```python
from build123d import *

# Parameters (mm, degrees)
SKETCH1_R      = 0.55
EXTRUDE1_DEPTH = 1


with BuildPart() as part:
    # Sketch1 → Extrude1 (new body)
    with BuildSketch(Plane.XY):
        with BuildLine():
            Line((1.656441889, -6.181925288), (2.174079979, -8.113776941))
            ThreePointArc((2.174079979, -8.113776941), (4.904287135, -6.819675043), (7, -4.643274706))
            Line((7, -4.643274706), (7, -3.161966685))
            ThreePointArc((7, -3.161966685), (0, 8.4), (-7, -3.161966685))
            Line((-7, -3.161966685), (-7, -4.643274706))
            ThreePointArc((-7, -4.643274706), (-4.904287135, -6.819675043), (-2.174079979, -8.113776941))
            Line((-2.174079979, -8.113776941), (-1.656441889, -6.181925288))
            ThreePointArc((-1.656441889, -6.181925288), (0, 6.4), (1.656441889, -6.181925288))
        make_face()
        with Locations((-2.86, -6.809962004)):
            Circle(SKETCH1_R, mode=Mode.SUBTRACT)
        with Locations(Location((2.86, -6.809962004, 0), (0, 0, 180))):
            Circle(SKETCH1_R, mode=Mode.SUBTRACT)
    extrude(amount=EXTRUDE1_DEPTH)


solid = part.part
```
Geometry check sheet. Reference: the model listing, model coordinates, mm. A direction names the side the tool comes from. Round coordinates to 2 decimals unless told otherwise and drop trailing zeros. Loops run counter-clockwise (first coordinate to the right, second up) from the corner with the lowest first, then second, coordinate; pieces in that order, holes last. Notation, with made-up numbers: (-14.75, -15.75) - (-3.75, -15.75) arc R14 cw to (-3.75, 11.25) - close; hole circle Ø5 at (-21, 30). An arc over 180 degrees is marked (long way). Write each question's results on one line, items separated by ' | '. Start each with the question number.
Q1. Thickness scan on line 1 (Y direction, x = -2.86, z = 0.5); line 2 (X direction, y = -7.25, z = 0.4); line 3 (X direction, y = 0.25, z = 0.3). Record the ranges inside material, lowest first. Write a range as [from, to].
Q2. Access from +Z, -Z, +X, -X, +Y, -Y to the whole of each face (thin tool, end or side, straight path). Record for faces 1 (the cylindrical face through (2.61, -6.32, 0.49)), 2 (the flat face through (-1.92, -7.16, 0.49)), 3 (the flat face through (7, -3.9, 0.5)).
Q3. Cross-section at D-D on y = 3.5. Enter the section's corners in (x, z).
Q4. Cross-section at C-C on z = 0.45. Enter the section's corners in (x, y), and give its area (3 significant figures).
Q5. Gauge pin test, flat ends, axial feed: P1, Ø1, axis at x = 2.86, y = -6.81, coming from the +Z side; P2, Ø0.5, axis at y = -4, z = 0.5, coming from the +X side. Record the tip position at first contact, or that the pin passes through.
Q6. Cross-section at B-B on y = 0.5. Enter the section's corners in (x, z), and give its area (3 significant figures).
Q7. Release check for a two-part mould opening along X. For faces 4 (the flat face through (-1.8, 6.3, 1)), 5 (the cylindrical face through (-2.61, -7.3, 0.49)), 6 (the flat face through (-7, -3.9, 0.5)) record: +X half, -X half, draft (parallel to the pull), parting line (faces both ways), or undercut.
Q8. Cross-section at A-A on x = -2.75. Enter the section's corners in (y, z).
Answers below:
1) line 1: y = [-7.9, -7.36], [-6.26, -5.73], [5.73, 7.86] | line 2: x = [-4.24, -3.19], [-2.53, -1.94], [1.94, 2.53], [3.19, 4.24] | line 3: x = [-7.9, -6.4], [6.4, 7.9]
2) face 1: +Z, -Z | face 2: +Z, -Z, -Y | face 3: +Z, -Z, +X, -Y
3) outline: (-7.31, 0) - (-5.36, 0) - (-5.36, 1) - (-7.31, 1) - close; (5.36, 0) - (7.31, 0) - (7.31, 1) - (5.36, 1) - close
4) outline: (-7, -4.64) arc R8.4 ccw to (-2.17, -8.11) - (-1.66, -6.18) arc R6.4 cw (long way) to (1.66, -6.18) - (2.17, -8.11) arc R8.4 ccw to (7, -4.64) - (7, -3.16) arc R7.9 ccw (long way) to (-7, -3.16) - close; hole circle Ø1.1 at (-2.86, -6.81); hole circle Ø1.1 at (2.86, -6.81) | area: 73.2 mm²
5) P1: passes through | P2: stops at x = 7
6) outline: (-7.9, 0) - (-6.38, 0) - (-6.38, 1) - (-7.9, 1) - close; (6.38, 0) - (7.9, 0) - (7.9, 1) - (6.38, 1) - close | area: 3.04 mm²
7) face 4: draft | face 5: undercut | face 6: -X half
8) outline: (-7.94, 0) - (-7.35, 0) - (-7.35, 1) - (-7.94, 1) - close; (-6.27, 0) - (-5.78, 0) - (-5.78, 1) - (-6.27, 1) - close; (5.78, 0) - (7.91, 0) - (7.91, 1) - (5.78, 1) - close
